Design review of the part shown in the three views and the two pictorial views. Dimensions are in mm from the part's minimum x, y and z. Round coordinates to 2 decimals unless told otherwise and drop trailing zeros. Order: outer loops, then holes, each group sorted by start corner. A loop starts at its lowest first (then second) coordinate and runs counter-clockwise, first axis right, second up.
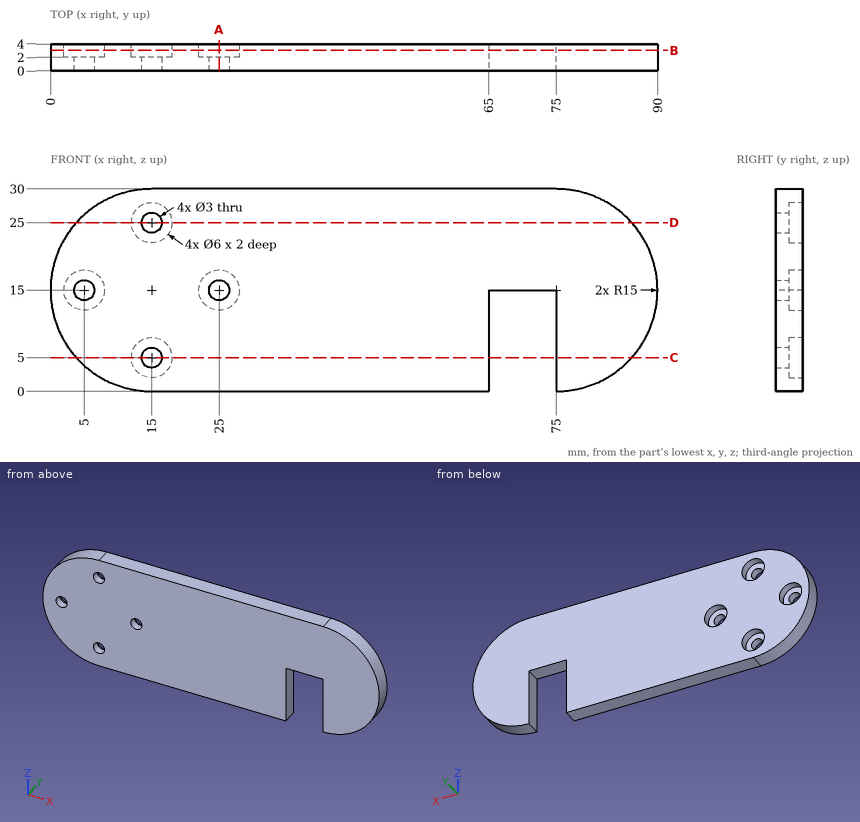
1) Take a section at D-D on z = 25. Give the boundary of the cut face in (x, y).
Results:
outline: (3.82, 0) - (13.5, 0) - (13.5, 2) - (12, 2) - (12, 4) - (3.82, 4) - close; (16.5, 0) - (86.18, 0) - (86.18, 4) - (18, 4) - (18, 2) - (16.5, 2) - close
2) To check wall thickness, follow line 1 along Z through (x, y) = (15, 0.55); line 2 along Z through (x, y) = (68, 0.85); line 3 along X through (y, z) = (0.8, 16). State the ranges of each line that lie inside material, in increasing order.
Results:
line 1: z = 0 to 3.5, 6.5 to 23.5, 26.5 to 30
line 2: z = 15 to 30
line 3: x = 0.03 to 3.88, 6.12 to 23.88, 26.12 to 89.97
3) Take a section at C-C on z = 5. Give the boundary of the cut face in (x, y).
Results:
outline: (3.82, 0) - (13.5, 0) - (13.5, 2) - (12, 2) - (12, 4) - (3.82, 4) - close; (16.5, 0) - (65, 0) - (65, 4) - (18, 4) - (18, 2) - (16.5, 2) - close; (75, 0) - (86.18, 0) - (86.18, 4) - (75, 4) - close
4) Take a section at A-A on x = 25. Give the boundary of the cut face in (y, z).
Results:
outline: (0, 0) - (4, 0) - (4, 12) - (2, 12) - (2, 13.5) - (0, 13.5) - close; (0, 16.5) - (2, 16.5) - (2, 18) - (4, 18) - (4, 30) - (0, 30) - close
5) Clearance check with flat-ended pins moving along their axes: P1, Ø1.5, axis at y = 1, z = 21.5, coming from the +X side; P2, Ø1.2, axis at x = 70.5, y = 2.5, coming from the -Z side; P3, Ø3, axis at x = 4.5, z = 15, coming from the +Y side. State where each tip first meets the part, or that it passes through.
Results:
P1: stops at x = 88.85
P2: stops at z = 15
P3: stops at y = 2
6) Take a section at B-B on y = 3.05. Give the boundary of the cut face in (x, z), plus the area to 3 significant figures.
Results:
outline: (15, 0) - (65, 0) - (65, 15) - (75, 15) - (75, 0) arc R15 ccw to (75, 30) - (15, 30) arc R15 ccw to start; hole circle Ø6 at (5, 15); hole circle Ø6 at (15, 5); hole circle Ø6 at (15, 25); hole circle Ø6 at (25, 15)
area: 2,240 mm2
